Here's how the part is built. I have some questions about the finished solid (model axes, mm). Round coordinates to 2 decimals unless told otherwise and drop trailing zeros. Answer in a Markdown table with one row per item.
```python
from build123d import *

# Parameters (mm, degrees)
SKETCH1_W           = 4
SKETCH1_H           = 8
SKETCH1_R           = 1.5
SKETCH1_R_2         = 1.4
BOSS_EXTRUDE2_DEPTH = 4


with BuildPart() as part:
    # Sketch1 → Boss-Extrude2 (new body)
    with BuildSketch(Plane.XY):
        Polygon((-10, 80), (-60, 80), (-60, -80), (60, -80), (60, 80), (10, 80), align=None)
        with Locations((-55, -66)):
            Rectangle(SKETCH1_W, SKETCH1_H, mode=Mode.SUBTRACT)
        with Locations((-55, -49.5)):
            Circle(SKETCH1_R, mode=Mode.SUBTRACT)
        with Locations((-10, -70)):
            Circle(SKETCH1_R, mode=Mode.SUBTRACT)
        with Locations((-55, -33)):
            Rectangle(SKETCH1_W, SKETCH1_H, mode=Mode.SUBTRACT)
        with Locations((10, -70)):
            Circle(SKETCH1_R, mode=Mode.SUBTRACT)
        with Locations((55, -66)):
            Rectangle(SKETCH1_W, SKETCH1_H, mode=Mode.SUBTRACT)
        with Locations((55, -49.5)):
            Circle(SKETCH1_R, mode=Mode.SUBTRACT)
        with Locations((55, -33)):
            Rectangle(SKETCH1_W, SKETCH1_H, mode=Mode.SUBTRACT)
        with Locations((-55, 0)):
            Circle(SKETCH1_R, mode=Mode.SUBTRACT)
        with Locations((-55, 33)):
            Rectangle(SKETCH1_W, SKETCH1_H, mode=Mode.SUBTRACT)
        with Locations((-19, 15.8)):
            Circle(SKETCH1_R_2, mode=Mode.SUBTRACT)
        with Locations((-55, 49.5)):
            Circle(SKETCH1_R, mode=Mode.SUBTRACT)
        with Locations((-55, 66)):
            Rectangle(SKETCH1_W, SKETCH1_H, mode=Mode.SUBTRACT)
        with Locations((-19, 54.8)):
            Circle(SKETCH1_R_2, mode=Mode.SUBTRACT)
        with Locations((19, 15.8)):
            Circle(SKETCH1_R_2, mode=Mode.SUBTRACT)
        with Locations((55, 0)):
            Circle(SKETCH1_R, mode=Mode.SUBTRACT)
        with Locations((55, 33)):
            Rectangle(SKETCH1_W, SKETCH1_H, mode=Mode.SUBTRACT)
        with Locations((19, 54.8)):
            Circle(SKETCH1_R_2, mode=Mode.SUBTRACT)
        with Locations((55, 49.5)):
            Circle(SKETCH1_R, mode=Mode.SUBTRACT)
        with Locations((55, 66)):
            Rectangle(SKETCH1_W, SKETCH1_H, mode=Mode.SUBTRACT)
    extrude(amount=BOSS_EXTRUDE2_DEPTH)


solid = part.part
```
1. For pin 1 Ø2.5 at (x, y) = (55, 0) entering from +Z, with a flat end and sliding along its axis, tell me the tip position at first contact or that it passes through.
Numbers:
| item | result |
|---|---|
| pin 1 | passes through |
2. Please list where these lines run through material, in increasing order: line 1 along X through (y, z) = (-31.5, 0.9); line 2 along Y through (x, z) = (-19, 3.15); line 3 along X through (y, z) = (-71, 2.8).
Numbers:
| item | result |
|---|---|
| line 1 | x = -60 to -57, -53 to 53, 57 to 60 |
| line 2 | y = -80 to 14.4, 17.2 to 53.4, 56.2 to 80 |
| line 3 | x = -60 to -11.12, -8.88 to 8.88, 11.12 to 60 |
3. Suppose I cut it at A-A on z = 1.1. State how many separate pieces and enclosed holes the cut face has, then the cut area to 3 significant figures.
Numbers:
| item | result |
|---|---|
| separate pieces | 1 |
| enclosed holes | 20 |
| area | 18,900 mm2 |
4. We'd pull the mould along Y, two halves only. Please class faces 1 (the face through (-55, 62, 2)), 2 (the face through (-60, 1, 2)): released by +Y, released by -Y, zero draft, split by the parting line, or undercut.
Numbers:
| item | result |
|---|---|
| face 1 | undercut |
| face 2 | zero draft |
